```python
from build123d import *

# Parameters (mm, degrees)
SKETCH003_R     = 13
SKETCH003_R_2   = 5.95
PAD001_DEPTH    = 20
SKETCH004_R     = 13
SKETCH004_R_2   = 6.25
POCKET001_DEPTH = 19


with BuildPart() as coil:
    # Sketch003 → Pad001 (new body)
    with BuildSketch(Plane.XY):
        Circle(SKETCH003_R)
        Circle(SKETCH003_R_2, mode=Mode.SUBTRACT)
    extrude(amount=PAD001_DEPTH)

    # Sketch004 → Pocket001 (cut)
    with BuildSketch(Plane.XY):
        Circle(SKETCH004_R)
        Circle(SKETCH004_R_2, mode=Mode.SUBTRACT)
    extrude(amount=POCKET001_DEPTH, mode=Mode.SUBTRACT)


with BuildPart() as coil001:
    # Body003 base: copy of coil
    add(coil.part)


with BuildPart() as coil001_1:
    # Body003 placement: moved
    add(coil001.part.moved(Location((0, 0, 20))))


with BuildPart() as coil002:
    # Body004 base: copy of coil001
    add(coil001_1.part)


with BuildPart() as coil002_1:
    # Clone001 placement: moved
    add(coil002.part.moved(Location((0, 0, -20))))


with BuildPart() as coil002_2:
    # Body004 placement: moved
    add(coil002_1.part.moved(Location((0, 0, 40))))


with BuildPart() as coil003:
    # Body005 base: copy of coil
    add(coil.part)


with BuildPart() as coil003_1:
    # Body005 placement: moved
    add(coil003.part.moved(Location((0, 0, 60))))


with BuildPart() as coil004:
    # Body006 base: copy of coil
    add(coil.part)


with BuildPart() as coil004_1:
    # Body006 placement: moved
    add(coil004.part.moved(Location((0, 0, 80))))


with BuildPart() as coil005:
    # Body012 base: copy of coil
    add(coil.part)


with BuildPart() as coil005_1:
    # Body012 placement: moved
    add(coil005.part.moved(Location((0, 0, 100))))


with BuildPart() as coilsfusion:
    # Fusion base: copy of coil
    add(coil.part)

    # Fusion: union coil001, coil002, coil003, coil004, coil005
    add(coil001_1.part)
    add(coil002_2.part)
    add(coil003_1.part)
    add(coil004_1.part)
    add(coil005_1.part)


solid = coilsfusion.part
```
Geometry check sheet. Reference: the model listing, model coordinates, mm. A direction names the side the tool comes from. Coordinates: 2 decimals unless noted, no trailing zeros. Order: outer loops, then holes, each group sorted by start corner. A loop starts at its lowest first (then second) coordinate and runs counter-clockwise, first axis right, second up.
Q1. Tool access check on faces 4 (the face through (-4.385, 4.021, 59.16)), 5 (the face through (6, 3, 100)). Record the directions out of +Z, -Z, +X, -X, +Y, -Y that give a thin tool (end or side, any length) a straight path to the whole face; none if there is none.
Reply:
face 4: +Z, -Z
face 5: none
Q2. Sectioned sample at A-A on x = 10.75. Record the cut outline in (y, z), and give its area (3 significant figures).
Reply:
outline: (-7.31, 19) - (7.31, 19) - (7.31, 20) - (-7.31, 20) - close; (-7.31, 39) - (7.31, 39) - (7.31, 40) - (-7.31, 40) - close; (-7.31, 59) - (7.31, 59) - (7.31, 60) - (-7.31, 60) - close; (-7.31, 79) - (7.31, 79) - (7.31, 80) - (-7.31, 80) - close; (-7.31, 99) - (7.31, 99) - (7.31, 100) - (-7.31, 100) - close; (-7.31, 119) - (7.31, 119) - (7.31, 120) - (-7.31, 120) - close
area: 87.7 mm2
Q3. Sectioned sample at C-C on y = 11. Record the cut outline in (x, z).
Reply:
outline: (-6.93, 19) - (6.93, 19) - (6.93, 20) - (-6.93, 20) - close; (-6.93, 39) - (6.93, 39) - (6.93, 40) - (-6.93, 40) - close; (-6.93, 59) - (6.93, 59) - (6.93, 60) - (-6.93, 60) - close; (-6.93, 79) - (6.93, 79) - (6.93, 80) - (-6.93, 80) - close; (-6.93, 99) - (6.93, 99) - (6.93, 100) - (-6.93, 100) - close; (-6.93, 119) - (6.93, 119) - (6.93, 120) - (-6.93, 120) - close
Q4. Draft check along Z on faces 1 (the face through (6, -3, 120)), 2 (the face through (-10.316, -7.91, 59.493)), 3 (the face through (5.96, 1.88, 49.37)). Enter one of: released by +Z, released by -Z, zero draft, split by the parting line, or undercut.
Reply:
face 1: released by +Z
face 2: zero draft
face 3: undercut
Q5. Depth check by flat-ended pin: pin 1 Ø3 at (x, z) = (5, 100) entering from -Y; pin 2 Ø2 at (x, y) = (-5, -7.5) entering from -Z; pin 3 Ø8 at (x, z) = (-1, 71.5) entering from +Y; pin 4 Ø4 at (y, z) = (9.5, 103.5) entering from -X. Enter the tip coordinate at first touch or a pass-through.
Reply:
pin 1: stops at y = -12.52
pin 2: stops at z = 19
pin 3: stops at y = 6.25
pin 4: passes through
Q6. Sectioned sample at B-B on z = 62.5. Record the cut outline in (x, y).
Reply:
outline: circle Ø12.5 at (0, 0); hole circle Ø11.9 at (0, 0)
Q7. Thickness scan on probe 1 along Z at (x, y) = (9.75, -7.5); probe 2 along Y at (x, z) = (0, 53.5); probe 3 along Y at (x, z) = (-1.75, 65). Record the ranges inside material, lowest first.
Reply:
probe 1: z = 19 to 20, 39 to 40, 59 to 60, 79 to 80, 99 to 100, 119 to 120
probe 2: y = -6.25 to -5.95, 5.95 to 6.25
probe 3: y = -6 to -5.69, 5.69 to 6
